```python
from build123d import *

# Parameters (mm, degrees)
SKETCH1_W               = 6.485
SKETCH1_H               = 4.5
BOSS_EXTRUDE1_DEPTH     = 88
BOSS_EXTRUDE1_2_DEPTH   = 88
SKETCH3_W               = 2
SKETCH3_H               = 1.5
CUT_EXTRUDE2_DEPTH      = 30
SKETCH4_W               = 2
SKETCH4_H               = 4.5
CUT_EXTRUDE3_DEPTH      = 65
BOSS_EXTRUDE2_REACH     = 93.644
SKETCH6_W               = 67
SKETCH6_H               = 3
BOSS_EXTRUDE3_DEPTH     = 5
CUT_EXTRUDE4_DEPTH      = 5
BOSS_EXTRUDE4_DEPTH     = 5
BOSS_EXTRUDE5_START     = 7
BOSS_EXTRUDE5_DEPTH     = 48
BOSS_EXTRUDE6_DEPTH     = 48
FILLET1_R               = 11
SKETCH18_W              = 14.57033113
SKETCH18_H              = 3
BOSS_EXTRUDE7_DEPTH     = 7
SKETCH15_W              = 23.7
SKETCH15_H              = 21.22267295
CUT_EXTRUDE6_DEPTH      = 7
SKETCH16_W              = 16.7
SKETCH16_H              = 1.5
CUT_EXTRUDE7_DEPTH      = 19
CUT_EXTRUDE5_DEPTH      = 92.727000479
CUT_EXTRUDE5_DEPTH_BACK = 92.727000479
SKETCH13_R              = 1.5
SKETCH17_W              = 14
SKETCH17_H              = 55
CUT_EXTRUDE8_DEPTH      = 3


with BuildPart() as part:
    # Sketch1 → Boss-Extrude1 (new body)
    with BuildSketch(Plane.XY):
        with Locations((-11.5925, 2.25)):
            Rectangle(SKETCH1_W, SKETCH1_H)
    extrude(amount=-BOSS_EXTRUDE1_DEPTH)


with BuildPart() as body_2:
    # Sketch1 → Boss-Extrude1 2 (new body)
    with BuildSketch(Plane.XY):
        with Locations((11.5925, 2.25)):
            Rectangle(SKETCH1_W, SKETCH1_H)
    extrude(amount=-BOSS_EXTRUDE1_2_DEPTH)


with BuildPart() as cut_extrude2_tool:
    # Sketch3 → Cut-Extrude2 (new body)
    with BuildSketch(Plane.XY):
        with Locations((-9.35, 0.75)):
            Rectangle(SKETCH3_W, SKETCH3_H)
        with Locations((9.35, 0.75)):
            Rectangle(SKETCH3_W, SKETCH3_H)
    extrude(amount=-CUT_EXTRUDE2_DEPTH)


with BuildPart() as part_1:
    add(part.part)

    # Cut-Extrude2: cut by cut_extrude2_tool
    add(cut_extrude2_tool.part, mode=Mode.SUBTRACT)


with BuildPart() as body_2_1:
    add(body_2.part)

    # Cut-Extrude2: cut by cut_extrude2_tool
    add(cut_extrude2_tool.part, mode=Mode.SUBTRACT)


with BuildPart() as cut_extrude3_tool:
    # Sketch4 → Cut-Extrude3 (new body)
    with BuildSketch(Plane(origin=(0, 0, -88), x_dir=(-1, 0, 0), z_dir=(0, 0, -1))):
        with Locations((9.35, 2.25)):
            Rectangle(SKETCH4_W, SKETCH4_H)
        with Locations((-9.35, 2.25)):
            Rectangle(SKETCH4_W, SKETCH4_H)
    extrude(amount=-CUT_EXTRUDE3_DEPTH)


with BuildPart() as part_2:
    add(part_1.part)

    # Cut-Extrude3: cut by cut_extrude3_tool
    add(cut_extrude3_tool.part, mode=Mode.SUBTRACT)


with BuildPart() as body_2_2:
    add(body_2_1.part)

    # Cut-Extrude3: cut by cut_extrude3_tool
    add(cut_extrude3_tool.part, mode=Mode.SUBTRACT)

    # Boss-Extrude2: up to this face of the body (flat: up to its plane)
    boss_extrude2_end = Plane(body_2_2.part.faces().sort_by_distance((10.35, 2.091743119, -50.857798165))[0])
    # Sketch6 → Boss-Extrude2 (add, up to the picked face)
    with BuildSketch(Plane(origin=(-10.35, 0, 0), x_dir=(0, 0, -1), z_dir=(1, 0, 0)), mode=Mode.PRIVATE) as boss_extrude2_sk1:
        with Locations((49.5, 3)):
            Rectangle(SKETCH6_W, SKETCH6_H)
    boss_extrude2_tool1 = split(extrude(boss_extrude2_sk1.sketch, amount=BOSS_EXTRUDE2_REACH, mode=Mode.PRIVATE), bisect_by=boss_extrude2_end, keep=Keep.BOTH, mode=Mode.PRIVATE)

    add(part_2.part)  # Boss-Extrude2 merges part
    add(boss_extrude2_tool1.solids().sort_by(Axis((-10.35, 3, -49.5), (1, 0, 0)))[0])

    # Sketch8 → Boss-Extrude3 (add)
    with BuildSketch(Plane(origin=(0, 0, -88), x_dir=(-1, 0, 0), z_dir=(0, 0, -1))):
        Polygon((-14.835, 25.70767295), (-14.835, 4.5), (-10.35, 4.5), (-10.35, 21.22267295), (10.35, 21.22267295), (10.35, 4.5), (14.835, 4.5), (14.835, 25.70767295), align=None)
    extrude(amount=-BOSS_EXTRUDE3_DEPTH)

    # Sketch9 → Cut-Extrude4 (cut)
    with BuildSketch(Plane(origin=(0, 0, -88), x_dir=(-1, 0, 0), z_dir=(0, 0, -1))):
        with BuildLine():
            Line((-15.009070225, 25.881743175), (-15.009070225, 22.527310239))
            ThreePointArc((-15.009070225, 22.527310239), (-13.436955933, 24.309628883), (-11.654637289, 25.881743175))
            Line((-11.654637289, 25.881743175), (-15.009070225, 25.881743175))
        make_face()
        with BuildLine():
            Line((15.009070225, 25.881743175), (15.009070225, 22.527310239))
            ThreePointArc((15.009070225, 22.527310239), (13.436955933, 24.309628883), (11.654637289, 25.881743175))
            Line((11.654637289, 25.881743175), (15.009070225, 25.881743175))
        make_face()
    extrude(amount=-CUT_EXTRUDE4_DEPTH, mode=Mode.SUBTRACT)

    # Sketch11 → Boss-Extrude4 (add)
    with BuildSketch(Plane.XY.offset(-83)):
        with BuildLine():
            Line((14.835, 4.5), (14.835, 22.748097759))
            ThreePointArc((14.835, 22.748097759), (13.436955933, 24.309628883), (11.875424809, 25.70767295))
            Line((11.875424809, 25.70767295), (-11.875424809, 25.70767295))
            ThreePointArc((-11.875424809, 25.70767295), (-13.436955933, 24.309628883), (-14.835, 22.748097759))
            Line((-14.835, 22.748097759), (-14.835, 4.5))
            Line((-14.835, 4.5), (14.835, 4.5))
        make_face()
    extrude(amount=BOSS_EXTRUDE4_DEPTH)

    # Sketch12 → Boss-Extrude5 (add)
    with BuildSketch(Plane.XY.offset(-78).offset(BOSS_EXTRUDE5_START)):
        Polygon((-14.835, 4.5), (-11.835, 7.5), (11.835, 7.5), (14.835, 4.5), align=None)
    extrude(amount=BOSS_EXTRUDE5_DEPTH)

    # Sketch14 → Boss-Extrude6 (add)
    with BuildSketch(Plane.XY.offset(-23)):
        Polygon((-11.835, 7.5), (-14.835, 4.5), (-10.835, 4.5), (-10.835, 7.5), align=None)
        Polygon((11.835, 7.5), (14.835, 4.5), (10.835, 4.5), (10.835, 7.5), align=None)
    extrude(amount=-BOSS_EXTRUDE6_DEPTH)

    # Fillet1
    # the kernel refuses this fillet: 11 mm, written as the material it takes off along each edge
    with BuildSketch(Plane(origin=(11.835, 7.5, -82.374586088), x_dir=(-1, 0, 0), z_dir=(0, 0, 1))) as fillet1_piece_1_section:
        with BuildLine():
            CenterArc((4.549834435, 11), FILLET1_R, 226.658241773, 43.341758227)
            Line((-3, 3), (0, 0))
            Line((0, 0), (4.549834435, 0))
        make_face()
    fillet1_piece_1 = extrude(amount=70.749172176, mode=Mode.PRIVATE)
    fillet1_piece_1 = split(fillet1_piece_1, bisect_by=Plane(origin=(11.355308805, 6.742969198, -78), z_dir=(0, 0, 1)), keep=Keep.TOP, mode=Mode.PRIVATE)
    add(fillet1_piece_1, mode=Mode.SUBTRACT)
    with BuildSketch(Plane(origin=(-11.835, 7.5, -82.374586088), x_dir=(1, 0, 0), z_dir=(0, 0, 1))) as fillet1_piece_2_section:
        with BuildLine():
            CenterArc((4.549834435, -11), FILLET1_R, 90, 43.341758227)
            Line((-3, -3), (0, 0))
            Line((0, 0), (4.549834435, 0))
        make_face()
    fillet1_piece_2 = extrude(amount=70.749172176, mode=Mode.PRIVATE)
    fillet1_piece_2 = split(fillet1_piece_2, bisect_by=Plane(origin=(-11.355308805, 6.742969198, -78), z_dir=(0, 0, 1)), keep=Keep.TOP, mode=Mode.PRIVATE)
    add(fillet1_piece_2, mode=Mode.SUBTRACT)

    # Sketch18 → Boss-Extrude7 (add)
    with BuildSketch(Plane(origin=(0, 0, -71), x_dir=(-1, 0, 0), z_dir=(0, 0, -1))):
        with Locations((0, 6)):
            Rectangle(SKETCH18_W, SKETCH18_H)
    extrude(amount=BOSS_EXTRUDE7_DEPTH)

    # Sketch15 → Cut-Extrude6 (cut)
    with BuildSketch(Plane(origin=(0, 0, -88), x_dir=(-1, 0, 0), z_dir=(0, 0, -1))):
        with Locations((0, 12.111336475)):
            Rectangle(SKETCH15_W, SKETCH15_H)
    extrude(amount=-CUT_EXTRUDE6_DEPTH, mode=Mode.SUBTRACT)

    # Sketch16 → Cut-Extrude7 (cut)
    with BuildSketch(Plane.XY):
        with BuildLine():
            ThreePointArc((11.5925, 3.75), (10.014054255, 3.189942939), (8.35, 3))
            Line((8.35, 3), (8.35, 4.5))
            Line((8.35, 4.5), (14.835, 4.5))
            ThreePointArc((14.835, 4.5), (13.170945745, 4.310057061), (11.5925, 3.75))
        make_face()
        with BuildLine():
            ThreePointArc((-11.5925, 3.75), (-10.014054255, 3.189942939), (-8.35, 3))
            Line((-8.35, 3), (-8.35, 4.5))
            Line((-8.35, 4.5), (-14.835, 4.5))
            ThreePointArc((-14.835, 4.5), (-13.170945745, 4.310057061), (-11.5925, 3.75))
        make_face()
        with Locations((0, 3.75)):
            Rectangle(SKETCH16_W, SKETCH16_H)
    extrude(amount=-CUT_EXTRUDE7_DEPTH, mode=Mode.SUBTRACT)

    # Sketch13 → Cut-Extrude5 (cut, two sides: drawn at the far end of the back side and taken through both)
    with BuildSketch(Plane(origin=(0, 4.5, 0), x_dir=(1, 0, 0), z_dir=(0, 1, 0)).offset(-CUT_EXTRUDE5_DEPTH_BACK)):
        with Locations(Location((10.542662348, 74.5, 0), (0, 0, 97.379545614))):
            Circle(SKETCH13_R)
        with Locations(Location((-10.542662348, 74.5, 0), (0, 0, 277.379545614))):
            Circle(SKETCH13_R)
        with Locations(Location((10.542662348, 21, 0), (0, 0, 97.379545614))):
            Circle(SKETCH13_R)
        with Locations(Location((-10.542662348, 21, 0), (0, 0, 277.379545614))):
            Circle(SKETCH13_R)
    extrude(amount=CUT_EXTRUDE5_DEPTH + CUT_EXTRUDE5_DEPTH_BACK, mode=Mode.SUBTRACT)

    # Sketch17 → Cut-Extrude8 (cut)
    with BuildSketch(Plane(origin=(0, 1.5, 0), x_dir=(-1, 0, 0), z_dir=(0, -1, 0))):
        with Locations((0, 53.5)):
            Rectangle(SKETCH17_W, SKETCH17_H)
    extrude(amount=-CUT_EXTRUDE8_DEPTH, mode=Mode.SUBTRACT)


solid = body_2_2.part
```
CAD build for the part. Positions are in the model's coordinates, mm. A direction names the side the tool comes from. Give positions to 0.01 mm unless a question says otherwise; leave off trailing zeros. Loops run counter-clockwise (first coordinate to the right, second up) from the corner with the lowest first, then second, coordinate; pieces in that order, holes last. Notation, with made-up numbers: M 73.5,53.25 L 87.5,53.25 A29 ccw 87.5,80.25 Z; hole C 57,-23.75 d8. An arc over 180 degrees is marked long. Use one line per item in the form item = value.
Item 1: Slice it at D-D (x = -2.75). List the corners of the cut face in (y, z), plus the area to 3 significant figures.
Determined:
outline = M 1.5,-26 L 4.5,-26 L 4.5,-81 L 22.72,-81 L 22.72,-88 L 25.71,-88 L 25.71,-78 L 7.5,-78 L 7.5,-23 L 4.5,-23 L 4.5,-19 L 3,-19 L 3,-16 L 1.5,-16 Z
area = 275 mm2
Item 2: Drill centre lines: probe 1 along X at (y, z) = (3.4, -74.5) (3 decimals); probe 2 along X at (y, z) = (3.3, -21) (3 decimals); probe 3 along X at (y, z) = (2.5, -61.5) (3 decimals). Where is each one in solid material? Low to high. Write a range as from..to.
Determined:
probe_1 = -14.835..-12.043, -9.043..-7, 7..9.043, 12.043..14.835
probe_2 = -14.835..-12.043, -9.043..9.043, 12.043..14.835
probe_3 = -14.835..-7, 7..14.835
Item 3: Flat gauge pins, fed straight in: pin 1 (3 mm diameter, centred on x = -4, y = 15.5, fed in from +Z); pin 2 (2.5 mm diameter, centred on x = -2, z = -17, fed in from +Y); pin 3 (7 mm diameter, centred on x = -0.5, z = -47, fed in from -Y). Where does each tip first touch, or does it go through?
Determined:
pin_1 = -78
pin_2 = 3
pin_3 = 4.5
Item 4: Which spindle directions (+Z, -Z, +X, -X, +Y, -Y) get a long thin tool onto all of the face, cutting with end or side? Do faces 4 (the face through (-12, 4.5, -73.7)), 5 (the face through (-7, 3, -53)), 6 (the face through (10.35, 1, -10)), 7 (the face through (-8.35, 2, -8)), 8 (the face through (0, 4.5, -21)). Say none if no direction does.
Determined:
face_4 = -X, +Y
face_5 = -Z, -Y
face_6 = +Z, -Z, -Y
face_7 = +Z, +Y, -Y
face_8 = +Z, +X, -X, +Y
Item 5: Slice it at C-C (y = 12.75). List the corners of the cut face in (x, z) (3 decimals).
Determined:
outline = M -14.835,-88 L -11.85,-88 L -11.85,-81 L 11.85,-81 L 11.85,-88 L 14.835,-88 L 14.835,-78 L -14.835,-78 Z
Item 6: Slice it at A-A (z = -21). List the corners of the cut face in (x, y) (3 decimals), plus the area to 3 significant figures.
Determined:
outline = M -14.835,0 L -12.043,0 L -12.043,4.5 L -14.835,4.5 Z; M -9.043,1.5 L 9.043,1.5 L 9.043,4.5 L -9.043,4.5 Z; M 12.043,0 L 14.835,0 L 14.835,4.5 L 12.043,4.5 Z
area = 79.4 mm2
Item 7: Two-plate mould, pull along X, no slides. Class faces 1 (the face through (11.4, 6.7, -47.3)), 2 (the face through (-10.35, 1, -82)), 3 (the face through (-11.293, 6.744, -47.336)): pulls with the +X half, pulls with the -X half, needs draft (parallel to the pull), parting line crosses it, or undercut.
Determined:
face_1 = pulls with the +X half
face_2 = undercut
face_3 = pulls with the -X half
